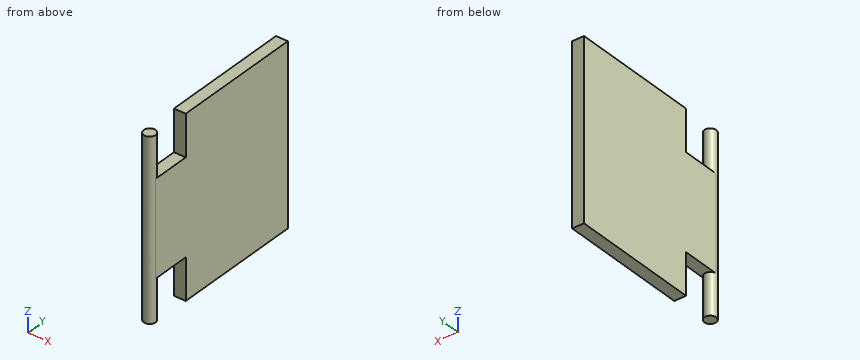
Autodesk Inventor part; units mm, degrees
ref_plane "YZ Plane" through (0, 0, 0) normal (1, 0, 0) x (0, 1, 0)
ref_plane "XZ Plane" through (0, 0, 0) normal (0, 1, 0) x (-1, 0, 0)
ref_plane "XY Plane" through (0, 0, 0) normal (0, 0, 1) x (1, 0, 0)
sketch "Sketch1" plane through (0, 0, 0) normal (0, 0, 1) x (1, 0, 0)
  circle A0 centre (0, 0) radius 1
  dimension "d0" = 2
extrude "Extrusion1" add sketch "Sketch1" along normal blind 30
ref_plane "Work Plane1" through (0, 0, 23) normal (0, 0, 1) x (1, 0, 0)
ref_plane "Work Plane2" through (0, 0, 7) normal (0, 0, -1) x (-1, 0, 0)
sketch "Sketch2" plane through (0, 0, 23) normal (0, 0, 1) x (1, 0, 0)
  circle A0 centre (0, 0) radius 1
  line L0 (1, 0) -> (-1, 0)
  line L1 (-1, 0) -> (-1, 28.5)
  line L2 (-1, 28.5) -> (1, 28.5)
  line L3 (1, 28.5) -> (1, 0)
  dimension "d7" = 28.5
extrude "Extrusion2" add sketch "Sketch2" against normal up to surface (16 mm away) contours A0 L1 L2 L3
sketch "Sketch3" plane through (1, 0, 23) normal (1, 0, 0) x (0, 0, -1)
  line L0 (16, 0) -> (16, 28.5)
  line L1 (0, 28.5) -> (16, 28.5)
  line L2 (0, 0) -> (0, 28.5)
  line L3 (16, 0) -> (0, 0)
  line L4 (0, 28.5) -> (-7, 28.5)
  line L5 (-7, 28.5) -> (-7, 6.5)
  line L6 (-7, 6.5) -> (0, 6.5)
  line L7 (0, 6.5) -> (0, 28.5)
  line L8 (16, 0) -> (16, 28.5)
  line L9 (16, 28.5) -> (23, 28.5)
  line L10 (23, 28.5) -> (23, 6.5)
  line L11 (23, 6.5) -> (16, 6.5)
  line L12 (16, 6.5) -> (16, 28.5)
  line L13 (23, -1) -> (23, 1)
  line L14 (-7, 1) -> (-7, -1)
  line L15 (16, 0) -> (0, 0)
  line L16 (16, 0) -> (16, 0)
  line L17 (16, 0) -> (0, 0)
  line L18 (0, 0) -> (0, 0)
  point P0 (23, 0)
  point P1 (19.5, 6.5)
  point P2 (-3.5, 6.5)
  point P3 (23, 0)
  point P4 (23, 17.5)
  point P5 (-7, 17.5)
  point P6 (-7, 0)
  dimension "d10" = 5.5
extrude "Extrusion3" add sketch "Sketch3" against normal up to surface (2 mm away) contours L0 L9 L10 L11 | L6 L5 L4 L2
properties part number "gpsDoor"
The listing builds one solid part. Answer for the finished solid, in the listing's coordinates (mm). Give positions to 0.01 mm unless a question says otherwise; leave off trailing zeros. Write each loop counter-clockwise with the first axis right and the second up, starting at its lowest first coordinate (ties: lowest second). Pieces come first, ordered by that corner, then holes.
1) Given P1, Ø1, axis at x = -0.5, y = 4, coming from the -Z side; P2, Ø1, axis at x = 0, y = 2, coming from the +Z side, each flat-ended and moving along its own axis, determine where each tip first touches the part or whether it passes through.
2) Section A-A (z = 26.75) is taken. Write down the section's boundary in (x, y), and give its area (3 significant figures).
3) Section B-B (x = 0) is taken. Write down the section's boundary in (y, z).
4) Section C-C (y = 2) is taken. Write down the section's boundary in (x, z), and give its area (3 significant figures).
5) Find the intervals of material crossed by L1, parallel to Y at x = -0.1, z = 28.5; L2, parallel to Y at x = -0.6, z = 3.75; L3, parallel to Y at x = -0.1, z = 14.5, in increasing order.
Response:
1. P1: stops at z = 7
1. P2: stops at z = 23
2. outline: circle Ø2 at (0, 0); (-1, 6.5) - (1, 6.5) - (1, 28.5) - (-1, 28.5) - close
2. area: 47.1 mm2
3. outline: (-1, 0) - (1, 0) - (1, 7) - (6.5, 7) - (6.5, 0) - (28.5, 0) - (28.5, 30) - (6.5, 30) - (6.5, 23) - (1, 23) - (1, 30) - (-1, 30) - close
4. outline: (-1, 7) - (1, 7) - (1, 23) - (-1, 23) - close
4. area: 32.0 mm2
5. L1: y = -0.99 to 0.99, 6.5 to 28.5
5. L2: y = -0.8 to 0.8, 6.5 to 28.5
5. L3: y = -0.99 to 28.5
